from build123d import *

# Parameters (mm, degrees)
BOSS_EXTRUDE1_DEPTH = 5.08
SKETCH4_W           = 29
SKETCH4_H           = 69
CUT_EXTRUDE1_DEPTH  = 5.08
SKETCH8_W           = 36.285714285
SKETCH8_H           = 5.08
SKETCH8_W_2         = 36.285714286
CUT_EXTRUDE2_DEPTH  = 5.08
SKETCH9_W           = 36.285714285
SKETCH9_H           = 5.08
SKETCH9_W_2         = 36.285714286
CUT_EXTRUDE3_DEPTH  = 5.08
SKETCH10_W          = 36.285714285
SKETCH10_H          = 5.08
SKETCH10_W_2        = 36.285714286
CUT_EXTRUDE4_DEPTH  = 5.08
SKETCH12_W          = 5.08
SKETCH12_H          = 6.35
CUT_EXTRUDE6_DEPTH  = 5.08


with BuildPart() as part:
    # Sketch1 → Boss-Extrude1 (new body)
    with BuildSketch(Plane(origin=(0, 0, 0), x_dir=(1, 0, 0), z_dir=(0, 1, 0))):
        Polygon((0, 0), (-254, 0), (-127, 219.970452561), align=None)
    extrude(amount=BOSS_EXTRUDE1_DEPTH)

    # Sketch4 → Cut-Extrude1 (cut)
    with BuildSketch(Plane(origin=(0, 5.08, 0), x_dir=(1, 0, 0), z_dir=(0, 1, 0))):
        with Locations((-189.76, 44.66)):
            Rectangle(SKETCH4_W, SKETCH4_H)
        with Locations((-64.24, 44.66)):
            Rectangle(SKETCH4_W, SKETCH4_H)
    extrude(amount=-CUT_EXTRUDE1_DEPTH, mode=Mode.SUBTRACT)

    # Sketch8 → Cut-Extrude2 (cut)
    with BuildSketch(Plane(origin=(-190.5, 0, -109.985226281), x_dir=(-0.5, 0, 0.866025404), z_dir=(-0.866025404, 0, -0.5))):
        with Locations((-72.571428572, 2.54)):
            Rectangle(SKETCH8_W, SKETCH8_H)
        with Locations((0, 2.54)):
            Rectangle(SKETCH8_W_2, SKETCH8_H)
        with Locations((72.571428572, 2.54)):
            Rectangle(SKETCH8_W, SKETCH8_H)
    extrude(amount=-CUT_EXTRUDE2_DEPTH, mode=Mode.SUBTRACT)

    # Sketch9 → Cut-Extrude3 (cut)
    with BuildSketch(Plane.XY):
        with Locations((-54.428571428, 2.54)):
            Rectangle(SKETCH9_W, SKETCH9_H)
        with Locations((-127, 2.54)):
            Rectangle(SKETCH9_W_2, SKETCH9_H)
        with Locations((-199.571428572, 2.54)):
            Rectangle(SKETCH9_W, SKETCH9_H)
    extrude(amount=-CUT_EXTRUDE3_DEPTH, mode=Mode.SUBTRACT)

    # Sketch10 → Cut-Extrude4 (cut)
    with BuildSketch(Plane(origin=(0, 0, 0), x_dir=(-0.5, 0, -0.866025404), z_dir=(0.866025404, 0, -0.5))):
        with Locations((54.428571428, 2.54)):
            Rectangle(SKETCH10_W, SKETCH10_H)
        with Locations((127, 2.54)):
            Rectangle(SKETCH10_W_2, SKETCH10_H)
        with Locations((199.571428572, 2.54)):
            Rectangle(SKETCH10_W, SKETCH10_H)
    extrude(amount=-CUT_EXTRUDE4_DEPTH, mode=Mode.SUBTRACT)

    # Sketch12 → Cut-Extrude6 (cut)
    with BuildSketch(Plane(origin=(0, 5.08, 0), x_dir=(1, 0, 0), z_dir=(0, 1, 0))):
        with Locations((-127, 165.995452561)):
            Rectangle(SKETCH12_W, SKETCH12_H)
    extrude(amount=-CUT_EXTRUDE6_DEPTH, mode=Mode.SUBTRACT)


solid = part.part
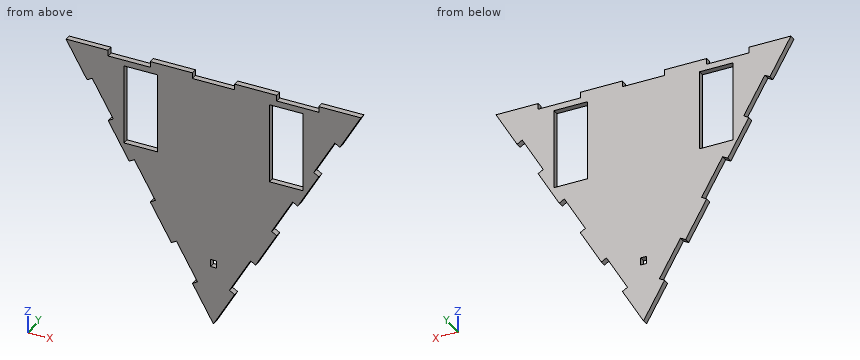
The listing builds one solid part. Answer for the finished solid, in the listing's coordinates (mm). Give positions to 0.01 mm unless a question says otherwise; leave off trailing zeros. Loops run counter-clockwise (first coordinate to the right, second up) from the corner with the lowest first, then second, coordinate; pieces in that order, holes last.
Item 1: A cutting plane is placed at B-B (y = 2.35). Give the number of separate pieces and of enclosed holes in the cut face, then the cut area to 3 significant figures.
Derived:
separate pieces: 1
enclosed holes: 3
area: 22,200 mm2
Item 2: A cutting plane is placed at A-A (z = -35). Give the vertices of the cut face in (x, y).
Derived:
outline: (-227.93, 0) - (-204.26, 0) - (-204.26, 5.08) - (-227.93, 5.08) - close; (-175.26, 0) - (-78.74, 0) - (-78.74, 5.08) - (-175.26, 5.08) - close; (-49.74, 0) - (-26.07, 0) - (-26.07, 5.08) - (-49.74, 5.08) - close
Item 3: A cutting plane is placed at C-C (x = -153). Give the vertices of the cut face in (y, z).
Derived:
outline: (0, -164.78) - (5.08, -164.78) - (5.08, 0) - (0, 0) - close
Item 4: A cutting plane is placed at D-D (z = -136). Give the vertices of the cut face in (x, y).
Derived:
outline: (-175.48, 0) - (-78.52, 0) - (-78.52, 5.08) - (-175.48, 5.08) - close
Item 5: Find the intervals of material crossed by line 1 along X through (y, z) = (0.7, -57.5); line 2 along X through (y, z) = (3.15, -67); line 3 along Z through (x, y) = (-70, 2.8), in increasing order.
Derived:
line 1: x = -214.94 to -204.26, -175.26 to -78.74, -49.74 to -39.06
line 2: x = -215.32 to -204.26, -175.26 to -78.74, -49.74 to -38.68
line 3: z = -111.08 to -79.16, -10.16 to -5.08
Item 6: Each of these flat-tipped pins is pushed along its axis until it touches: pin 1 Ø1.5 at (y, z) = (2.5, -1.5) entering from -X; pin 2 Ø1.5 at (y, z) = (1.5, -2) entering from +X; pin 3 Ø1 at (y, z) = (4, -161) entering from +X. Where does it stop, or does it pass through?
Derived:
pin 1: stops at x = -253.57
pin 2: stops at x = -0.72
pin 3: stops at x = -98.53
